Autodesk Inventor part; units mm, degrees
ref_plane "YZ Plane" through (0, 0, 0) normal (1, 0, 0) x (0, 1, 0)
ref_plane "XZ Plane" through (0, 0, 0) normal (0, 1, 0) x (-1, 0, 0)
ref_plane "XY Plane" through (0, 0, 0) normal (0, 0, 1) x (1, 0, 0)
sketch "Sketch1" plane through (0, 0, 0) normal (0, 0, 1) x (1, 0, 0)
  line L0 (0, 6) -> (0, -6)
  line L1 (0, -6) -> (1.25, -6)
  line L2 (1.25, -6) -> (1.5, -5.75)
  line L3 (1.5, -5.75) -> (1.5, 3.9)
  line L4 (1.6, 4) -> (2.5, 4)
  line L5 (2.75, 4.25) -> (2.75, 5.75)
  line L6 (2.5, 6) -> (0, 6)
  arc A0 (1.6, 4) -> (1.5, 3.9) centre (1.6, 3.9) ccw
  line L7 (2.5, 6) -> (2.75, 5.75)
  line L8 (2.5, 4) -> (2.75, 4.25)
  point P0 (0, 0)
  point P1 (2.75, 4)
  point P2 (2.75, 6)
  point P3 (0, 0)
  dimension "d0" = 5.5
  dimension "d1" = 2
  dimension "d3" = 3
  dimension "d4" = 3.2
  dimension "d5" = 135
  dimension "d6" = 0.25
  dimension "d7" = 10
  dimension "d9" = 0.25
revolve "Revolution1" add sketch "Sketch1" angle 360 about axis through (0, 6, 0) along (0, -1, 0)
sketch "Sketch2" plane through (0, 6, 0) normal (0, 1, 0) x (1, 0, 0)
  line L0 (0, -1.1547) -> (-1, -0.5774)
  line L1 (-1, -0.5774) -> (-1, 0.5774)
  line L2 (-1, 0.5774) -> (0, 1.1547)
  line L3 (0, 1.1547) -> (1, 0.5774)
  line L4 (1, 0.5774) -> (1, -0.5774)
  line L5 (1, -0.5774) -> (0, -1.1547)
  point P0 (0, 0)
  point P1 (0, 0)
  dimension "d11" = 2
extrude "Extrusion1" cut sketch "Sketch2" against normal blind 1.5
thread "Thread1"
sketch "Sketch3" plane through (0, 0, 0) normal (1, 0, 0) x (0, 1, 0)
  line L0 (6, 1.1547) -> (5, 0.1547)
  line L1 (5, 0.1547) -> (6, 0.1547)
  line L2 (6, 0.1547) -> (6, 1.1547)
  line L3 (-1.4, 0) -> (8.4, 0)
  point P0 (0, 0)
  dimension "d18" = 1
revolve "Revolution2" cut sketch "Sketch3" angle 360 about axis through (0, -10, 0) along (0, 1, 0)
properties part number "Bolt_M3x0.35_10mm_LSH" material "Stainless Steel"
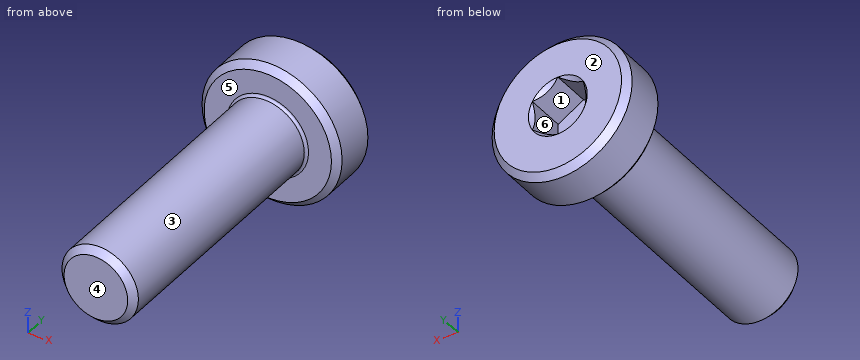
Verification items for the finished model (mm, model axes). Face numbers are marked on the shaded views. A direction names the side the tool comes from. Round coordinates to 2 decimals unless told otherwise and drop trailing zeros. Order: outer loops, then holes, each group sorted by start corner. A loop starts at its lowest first (then second) coordinate and runs counter-clockwise, first axis right, second up.
1. Release check for a two-part mould opening along Z. For the marked faces 1, 2 and 3 record: +Z half, -Z half, draft (parallel to the pull), parting line (faces both ways), or undercut.
Final values:
face 1: undercut
face 2: draft
face 3: parting line
2. Go/stop test with flat-tipped pins: P1, Ø1, axis at x = 0, z = 0, coming from the +Y side; P2, Ø1, axis at y = 0.5, z = 0, coming from the +X side; P3, Ø1.5, axis at y = -2, z = 1, coming from the -X side. Record where each tip stops, or that it passes through.
Final values:
P1: stops at y = 4.5
P2: stops at x = 1.5
P3: stops at x = -1.48
3. Thickness scan on L1, parallel to Y at x = 2.25, z = 0.65; L2, parallel to Y at x = 0.3, z = -0.6; L3, parallel to Z at x = 2.4, y = 5. Record the ranges inside material, lowest first.
Final values:
L1: y = 4 to 6
L2: y = -6 to 4.5
L3: z = -1.34 to 1.34
4. Access from +Z, -Z, +X, -X, +Y, -Y to the whole of each face (thin tool, end or side, straight path). Record for the marked faces 4, 5 and 6.
Final values:
face 4: +Z, -Z, +X, -X, -Y
face 5: -Y
face 6: +Y
5. Section check B-B on y = 1. Record the cut outline in (x, z), then the cut area to 3 significant figures.
Final values:
outline: circle Ø3 at (0, 0)
area: 7.07 mm2
6. Section check A-A on z = 0. Record the cut outline in (x, y).
Final values:
outline: (-2.75, 4.25) - (-2.5, 4) - (-1.6, 4) arc R0.1 cw to (-1.5, 3.9) - (-1.5, -5.75) - (-1.25, -6) - (1.25, -6) - (1.5, -5.75) - (1.5, 3.9) arc R0.1 cw to (1.6, 4) - (2.5, 4) - (2.75, 4.25) - (2.75, 5.75) - (2.5, 6) - (1.15, 6) - (1, 5.85) - (1, 4.5) - (-1, 4.5) - (-1, 5.85) - (-1.15, 6) - (-2.5, 6) - (-2.75, 5.75) - close
